```python
from build123d import *

# Parameters (mm, degrees)
F0_W     = 101.6
F0_H     = 50.8
F1_DEPTH = 76.2
F3_DEPTH = 25.4
F5_DEPTH = 25.4


with BuildPart() as f1:
    # F0 (on Front) → F1 (new body)
    with BuildSketch(Plane.XZ):
        with Locations((4.822348, -29.982933)):
            Rectangle(F0_W, F0_H)
    extrude(amount=F1_DEPTH)

    # F2 (on face) → F3 (join)
    with BuildSketch(Plane.XY.offset(-4.582933)):
        Polygon((30.222348, -76.2), (55.622348, -76.2), (55.622348, -38.1), align=None)
    extrude(amount=F3_DEPTH)

    # F4 (on face) → F5 (join)
    with BuildSketch(Plane.XY.offset(-4.582933)):
        Polygon((-45.977652, 0), (-45.977652, -76.2), (-20.577652, -76.2), (17.522348, 0), align=None)
    extrude(amount=F5_DEPTH)


solid = f1.part
```
Geometry check sheet. Reference: the model listing, model coordinates, mm. A direction names the side the tool comes from. Coordinates: 2 decimals unless noted, no trailing zeros. Order: outer loops, then holes, each group sorted by start corner. A loop starts at its lowest first (then second) coordinate and runs counter-clockwise, first axis right, second up. Notation, with made-up numbers: (-5, -32) - (45, -32) arc R20 ccw to (45, -5) - close; hole circle Ø5 at (-10, -6.5). An arc over 180 degrees is marked (long way). Answer as a JSON object with one key per item and string values. Group by question number.
Item 1: Sectioned sample at D-D, the plane y = -51. Record the cut outline in (x, z), and give its area (3 significant figures).
Item 2: Scan lines: probe 1 along Z at (x, y) = (13, -69.5); probe 2 along X at (y, z) = (-67, 16); probe 3 along X at (y, z) = (-54, 9). Record each from-to range of solid material in increasing order.
Item 3: Depth check by flat-ended pin: pin 1 Ø4 at (y, z) = (-18.5, 9.5) entering from +X. Enter the tip coordinate at first touch or a pass-through.
Item 4: Sectioned sample at A-A, the plane z = 6. Record the cut outline in (x, y).
Item 5: Sectioned sample at C-C, the plane x = 44. Record the cut outline in (y, z).
Item 6: Draft check along X on faces 1 (the face through (-45.978, -38, -18)), 2 (the face through (43.1, -56.88, 7.94)), 3 (the face through (4, -38, -55.383)). Enter one of: +X half, -X half, draft (parallel to the pull), parting line (faces both ways), or undercut.
Item 7: Tool access check on faces 4 (the face through (-1.794, -38.633, 7.939)), 5 (the face through (6, 0, -18)), 6 (the face through (25, -38, -4.583)). Record the directions out of +Z, -Z, +X, -X, +Y, -Y that give a thin tool (end or side, any length) a straight path to the whole face; none if there is none.
Item 8: Sectioned sample at B-B, the plane y = -65. Record the cut outline in (x, z).
Resolved:
{
 "1": {"outline": "(-45.98, -55.38) - (55.62, -55.38) - (55.62, 20.82) - (47.02, 20.82) - (47.02, -4.58) - (-7.98, -4.58) - (-7.98, 20.82) - (-45.98, 20.82) - close", "area": "6,340 mm^2"},
 "2": {"probe 1": "-55.38 to -4.58", "probe 2": "-45.98 to -15.98, 36.36 to 55.62", "probe 3": "-45.98 to -9.48, 45.02 to 55.62"},
 "3": {"pin 1": "x = 9.27"},
 "4": {"outline": "(-45.98, -76.2) - (-20.58, -76.2) - (17.52, 0) - (-45.98, 0) - close; (30.22, -76.2) - (55.62, -76.2) - (55.62, -38.1) - close"},
 "5": {"outline": "(-76.2, -55.38) - (0, -55.38) - (0, -4.58) - (-55.53, -4.58) - (-55.53, 20.82) - (-76.2, 20.82) - close"},
 "6": {"face 1": "-X half", "face 2": "undercut", "face 3": "draft"},
 "7": {"face 4": "+Z, -Y", "face 5": "+Z, -Z, +X, -X, +Y", "face 6": "+Z"},
 "8": {"outline": "(-45.98, -55.38) - (55.62, -55.38) - (55.62, 20.82) - (37.69, 20.82) - (37.69, -4.58) - (-14.98, -4.58) - (-14.98, 20.82) - (-45.98, 20.82) - close"}
}
